from build123d import *

# Parameters (mm, degrees)
SKETCH1_W           = 150
SKETCH1_H           = 130
SKETCH1_W_2         = 57
SKETCH1_H_2         = 106
BOSS_EXTRUDE1_DEPTH = 6
SKETCH2_R           = 2
CUT_EXTRUDE1_DEPTH  = 100.969995499


with BuildPart() as part:
    # Sketch1 → Boss-Extrude1 (new, symmetric)
    with BuildSketch(Plane(origin=(0, 0, 0), x_dir=(1, 0, 0), z_dir=(0, 1, 0))):
        Rectangle(SKETCH1_W, SKETCH1_H)
        with Locations((-34.5, 0)):
            Rectangle(SKETCH1_W_2, SKETCH1_H_2, mode=Mode.SUBTRACT)
        with Locations((34.5, 0)):
            Rectangle(SKETCH1_W_2, SKETCH1_H_2, mode=Mode.SUBTRACT)
    extrude(amount=BOSS_EXTRUDE1_DEPTH, both=True)

    # Sketch2 → Cut-Extrude1 (cut, through all)
    with BuildSketch(Plane(origin=(0, 6, 0), x_dir=(1, 0, 0), z_dir=(0, 1, 0))):
        with Locations(Location((-69, 0, 0), (0, 0, 270))):
            Circle(SKETCH2_R)
        with Locations(Location((69, 0, 0), (0, 0, 90))):
            Circle(SKETCH2_R)
        with Locations(Location((-10, -59, 0), (0, 0, 270))):
            Circle(SKETCH2_R)
        with Locations(Location((10, -59, 0), (0, 0, 90))):
            Circle(SKETCH2_R)
        with Locations(Location((-10, 59, 0), (0, 0, 90))):
            Circle(SKETCH2_R)
        with Locations(Location((10, 59, 0), (0, 0, 270))):
            Circle(SKETCH2_R)
    extrude(amount=-CUT_EXTRUDE1_DEPTH, mode=Mode.SUBTRACT)


solid = part.part
Input: part model. Units: mm. Frame: model coordinates. A direction names the side the tool comes from. Give positions to 0.01 mm unless a question says otherwise; leave off trailing zeros. Loops run counter-clockwise (first coordinate to the right, second up) from the corner with the lowest first, then second, coordinate; pieces in that order, holes last. Notation, with made-up numbers: M 32,45 L 67,45 A24 ccw 67,61 Z; hole C 28.5,39 d10. An arc over 180 degrees is marked long. Use one line per item in the form item = value.
1. Section query A-A, the plane x = 10. Return the cut outline in (y, z).
Numbers:
outline = M -6,-65 L 6,-65 L 6,-61 L -6,-61 Z; M -6,-57 L 6,-57 L 6,-53 L -6,-53 Z; M -6,53 L 6,53 L 6,57 L -6,57 Z; M -6,61 L 6,61 L 6,65 L -6,65 Z
2. Section query B-B, the plane z = -28.5. Return the cut outline in (x, y), and give its area (3 significant figures).
Numbers:
outline = M -75,-6 L -63,-6 L -63,6 L -75,6 Z; M -6,-6 L 6,-6 L 6,6 L -6,6 Z; M 63,-6 L 75,-6 L 75,6 L 63,6 Z
area = 432 mm²
3. Line query: L1, parallel to X at y = -3, z = -59; L2, parallel to X at y = 5.75, z = -43.5; L3, parallel to X at y = 3, z = 0. Output: solid intervals per line, ascending.
Numbers:
L1 = -75 to -12, -8 to 8, 12 to 75
L2 = -75 to -63, -6 to 6, 63 to 75
L3 = -75 to -71, -67 to -63, -6 to 6, 63 to 67, 71 to 75
4. Section query C-C, the plane x = 48. Return the cut outline in (y, z), and give its area (3 significant figures).
Numbers:
outline = M -6,-65 L 6,-65 L 6,-53 L -6,-53 Z; M -6,53 L 6,53 L 6,65 L -6,65 Z
area = 288 mm²
5. Reachability of faces 1 (the face through (-35, 0, 53)), 2 (the face through (-1, 6, -1)) from +Z, -Z, +X, -X, +Y, -Y: full face, straight path, thin tool, end or side. Return the list, or none.
Numbers:
face_1 = +Y, -Y
face_2 = +Z, -Z, +X, -X, +Y
6. First-contact query: pin 1 (2.5 mm diameter, centred on x = 10, z = -59, fed in from +Y). Flat tip, straight axial feed; report the tip coordinate or a pass-through.
Numbers:
pin_1 = through
7. Pull-direction query (Z, two-part tool) for faces 3 (the face through (-1, 0, 65)), 4 (the face through (63, 0, 1)), 5 (the face through (-75, 0, 1)), 6 (the face through (-1, 0, -65)); classes: released by +Z, released by -Z, zero draft, split by the parting line, or undercut.
Numbers:
face_3 = released by +Z
face_4 = undercut
face_5 = zero draft
face_6 = released by -Z
8. Section query D-D, the plane y = -4. Count the separate pieces of the cut face and the enclosed holes in it, and give its area (3 significant figures).
Numbers:
separate_pieces = 1
enclosed_holes = 8
area = 7,340 mm²
